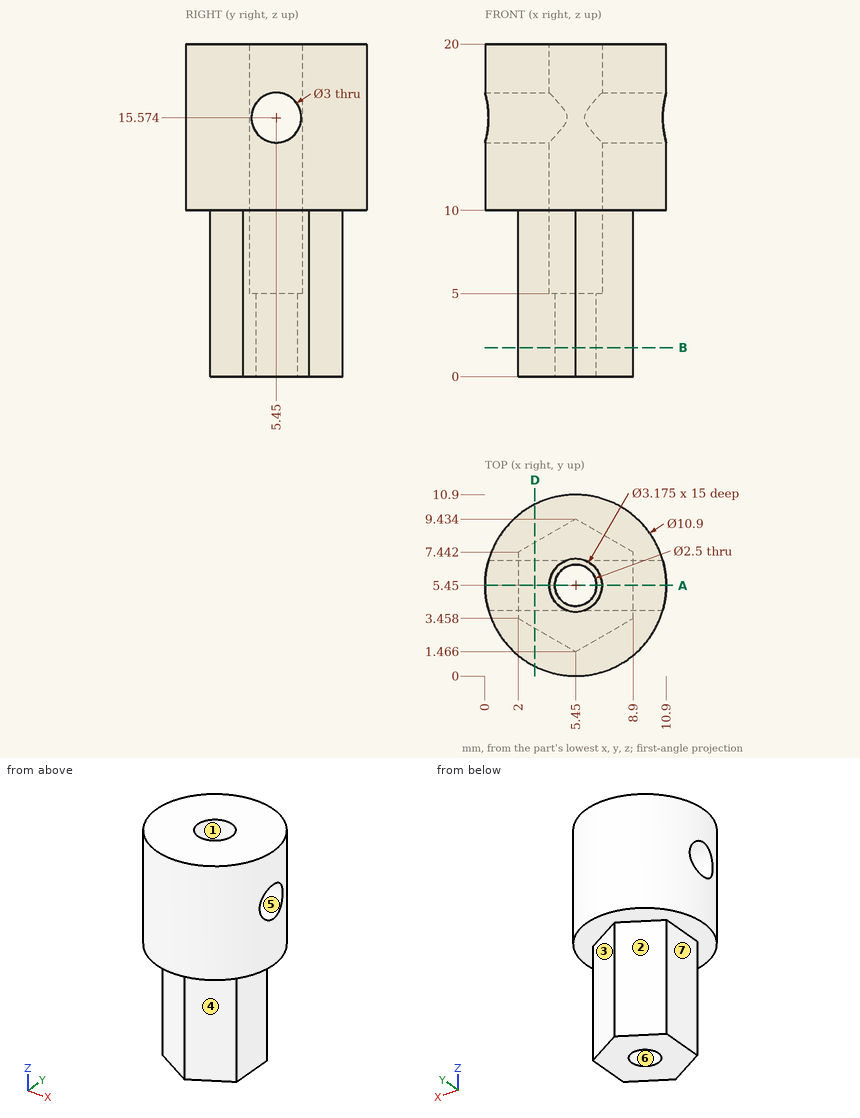
Input: dimensioned drawing with shaded views. Units: mm. Origin: part minimum x, y, z. A direction names the side the tool comes from. Coordinates: 2 decimals unless noted, no trailing zeros. Order: outer loops, then holes, each group sorted by start corner. A loop starts at its lowest first (then second) coordinate and runs counter-clockwise, first axis right, second up.
1. Draft query along X for the marked faces 4, 5, 6 and 7. Return one class per face: +X half, -X half, draft (parallel to the pull), parting line (faces both ways), or undercut.
Checked values:
face 4: +X half
face 5: draft
face 6: undercut
face 7: -X half
2. Cut plane A-A, the plane y = 5.45. Return loops of the section in (x, z).
Checked values:
outline: (0, 10) - (2, 10) - (2, 0) - (4.2, 0) - (4.2, 5) - (3.86, 5) - (3.86, 14.07) - (0, 14.07) - close; (0, 17.07) - (3.86, 17.07) - (3.86, 20) - (0, 20) - close; (6.7, 0) - (8.9, 0) - (8.9, 10) - (10.9, 10) - (10.9, 14.07) - (7.04, 14.07) - (7.04, 5) - (6.7, 5) - close; (7.04, 17.07) - (10.9, 17.07) - (10.9, 20) - (7.04, 20) - close
3. Cut plane B-B, the plane z = 1.75. Return loops of the section in (x, y).
Checked values:
outline: (2, 3.46) - (5.45, 1.47) - (8.9, 3.46) - (8.9, 7.44) - (5.45, 9.43) - (2, 7.44) - close; hole circle Ø2.5 at (5.45, 5.45)
4. Cut plane D-D, the plane x = 3. Return loops of the section in (y, z), plus the area to 3 significant figures.
Checked values:
outline: (0.58, 10) - (2.88, 10) - (2.88, 0) - (8.02, 0) - (8.02, 10) - (10.32, 10) - (10.32, 20) - (0.58, 20) - close; hole circle Ø3 at (5.45, 15.57)
area: 142 mm2
5. Ray query, line 1 along Z through (x, y) = (0.5, 5.5) (1 decimal); line 2 along Y through (x, z) = (5.5, 10.25); line 3 along Z through (x, y) = (2, 7.75). Return the intervals inside material, ascending.
Checked values:
line 1: z = 10 to 14.1, 17.1 to 20
line 2: y = 0 to 3.86, 7.04 to 10.9
line 3: z = 10 to 20
6. Contact query for flat-ended pins moving along their axis: P1, Ø4, axis at x = 9, z = 13, coming from the -Y side (1 decimal); P2, Ø5.5, axis at x = 8, y = 6, coming from the -Z side; P3, Ø6, axis at y = 2, z = 13, coming from the +X side; P4, Ø2, axis at x = 2, z = 12.5, coming from the +Y side. Output: stop coordinate, or through.
Checked values:
P1: stops at y = 0.2
P2: stops at z = 0
P3: stops at x = 10.88
P4: stops at y = 10.32
7. Access query for the marked faces 1, 2 and 3. Directions: +Z, -Z, +X, -X, +Y, -Y. A direction counts if a zero-diameter tool reaches every point of the face in a straight line with its end or side. Return the directions, or none.
Checked values:
face 1: +Z
face 2: -Z, -X, +Y
face 3: -Z, +X, +Y
